```python
from build123d import *

# Parameters (mm, degrees)
DODANIE_WYCI_GNI_CIE1_DEPTH = 30
WYTNIJ_WYCI_GNI_CIE1_REACH  = 54.202
SZKIC2_R                    = 2
SFAZOWANIE1_SIZE            = 8
SFAZOWANIE1_SIZE_2          = 18
SFAZOWANIE2_SIZE            = 8
SFAZOWANIE2_SIZE_2          = 18


with BuildPart() as part:
    # Szkic1 → Dodanie-wyciągnięcie1 (new body)
    with BuildSketch(Plane(origin=(0, 0, 0), x_dir=(1, 0, 0), z_dir=(0, 1, 0))):
        Polygon((-40, 0), (-27.5, -15), (27.5, -15), (40, 0), align=None)
    extrude(amount=DODANIE_WYCI_GNI_CIE1_DEPTH)

    # Szkic2 → Wytnij-wyciągnięcie1 (cut, up to next)
    with BuildSketch(Plane(origin=(0, 0, 0), x_dir=(-1, 0, 0), z_dir=(0, 0, -1)), mode=Mode.PRIVATE) as wytnij_wyci_gni_cie1_sk1:
        with Locations((-21, 15)):
            Circle(SZKIC2_R)
    wytnij_wyci_gni_cie1_tool1 = extrude(wytnij_wyci_gni_cie1_sk1.sketch, amount=-WYTNIJ_WYCI_GNI_CIE1_REACH, mode=Mode.PRIVATE) & part.part
    # Szkic2 → Wytnij-wyciągnięcie1 (cut, up to next)
    with BuildSketch(Plane(origin=(0, 0, 0), x_dir=(-1, 0, 0), z_dir=(0, 0, -1)), mode=Mode.PRIVATE) as wytnij_wyci_gni_cie1_sk2:
        with Locations((21, 15)):
            Circle(SZKIC2_R)
    wytnij_wyci_gni_cie1_tool2 = extrude(wytnij_wyci_gni_cie1_sk2.sketch, amount=-WYTNIJ_WYCI_GNI_CIE1_REACH, mode=Mode.PRIVATE) & part.part
    add(wytnij_wyci_gni_cie1_tool1.solids().sort_by_distance((21, 15, 0))[0], mode=Mode.SUBTRACT)
    add(wytnij_wyci_gni_cie1_tool2.solids().sort_by_distance((-21, 15, 0))[0], mode=Mode.SUBTRACT)

    # Sfazowanie1
    # the kernel refuses this chamfer: 18, 8 mm, written as the material it takes off along each edge
    with BuildSketch(Plane(origin=(-74.15058918, 0, 15), x_dir=(0, 0.996867139056945, 0.0790942922619672), z_dir=(1, 0, 0))) as sfazowanie1_piece_1:
        Polygon((SFAZOWANIE1_SIZE * 0.996867139057, -SFAZOWANIE1_SIZE * 0.079094292262), (-SFAZOWANIE1_SIZE_2 * 0.079094292262, -SFAZOWANIE1_SIZE_2 * 0.996867139057), (0, 0), align=None)
    extrude(amount=148.301178361, mode=Mode.SUBTRACT)

    # Sfazowanie2
    # the kernel refuses this chamfer: 18, 8 mm, written as the material it takes off along each edge
    with BuildSketch(Plane(origin=(-74.15058918, 30, 15), x_dir=(0, -0.996867139056945, 0.0790942922619672), z_dir=(1, 0, 0))) as sfazowanie2_piece_1:
        Polygon((SFAZOWANIE2_SIZE * 0.996867139057, SFAZOWANIE2_SIZE * 0.079094292262), (-SFAZOWANIE2_SIZE_2 * 0.079094292262, SFAZOWANIE2_SIZE_2 * 0.996867139057), (0, 0), align=None)
    extrude(amount=148.301178361, mode=Mode.SUBTRACT)


solid = part.part
```
Work out the finished part from the listing and answer in its coordinate system (mm). Give positions to 0.01 mm unless a question says otherwise; leave off trailing zeros. Write each loop counter-clockwise with the first axis right and the second up, starting at its lowest first coordinate (ties: lowest second). Pieces come first, ordered by that corner, then holes.
(1) The part is cut by section B-B on z = 6. Write down the section's boundary in (x, y).
Final values:
outline: (-35, 4) - (35, 4) - (35, 26) - (-35, 26) - close; hole circle Ø4 at (-21, 15); hole circle Ø4 at (21, 15)
(2) The part is cut by section A-A on x = 21. Write down the section's boundary in (y, z).
Final values:
outline: (1.33, 0) - (13, 0) - (13, 15) - (8, 15) - close; (17, 0) - (28.67, 0) - (22, 15) - (17, 15) - close
(3) Straight lines are drawn through the part: line 1 (X direction, y = 14, z = 9.75) (3 decimals); line 2 (Y direction, x = 21, z = 3.5); line 3 (Y direction, x = -21, z = 9.25). For each, find the intervals that lie inside material, in ascending order.
Final values:
line 1: x = -31.875 to -22.732, -19.268 to 19.268, 22.732 to 31.875
line 2: y = 2.89 to 13, 17 to 27.11
line 3: y = 5.44 to 13, 17 to 24.56
(4) The part is cut by section D-D on x = -8. Write down the section's boundary in (y, z).
Final values:
outline: (1.33, 0) - (28.67, 0) - (22, 15) - (8, 15) - close
(5) Flat-ended cylindrical pins translate along their axes: pin 1 Ø4 at (y, z) = (7.5, 9) entering from -X; pin 2 Ø2 at (x, y) = (-30.5, 23) entering from +Z; pin 3 Ø5 at (x, z) = (7.5, 13) entering from +Y; pin 4 Ø3 at (x, y) = (21, 15) entering from -Z. Find the tip coordinate at first contact, or state that the pin passes through.
Final values:
pin 1: stops at x = -34.17
pin 2: stops at z = 12.6
pin 3: stops at y = 24
pin 4: passes through
(6) The mould has two halves that part along Y. Classify faces 1 (the cylindrical face through (21, 17, 7)), 2 (the flat face through (1, 15, 0)), 3 (the flat face through (-0.56, 25.29, 7.6)), 4 (the cylindrical face through (-21, 17, 7)): pulls with the +Y half, pulls with the -Y half, needs draft (parallel to the pull), parting line crosses it, or undercut.
Final values:
face 1: undercut
face 2: needs draft
face 3: pulls with the +Y half
face 4: undercut
(7) The part is cut by section C-C on y = 8.75. Write down the section's boundary in (x, z).
Final values:
outline: (-40, 0) - (40, 0) - (27.5, 15) - (-27.5, 15) - close
